```python
from build123d import *

# Parameters (mm, degrees)
SKETCH2_R           = 2.65
BOSS_EXTRUDE1_DEPTH = 2
SKETCH3_R           = 4
BOSS_EXTRUDE2_DEPTH = 10


with BuildPart() as part:
    # Sketch2 → Boss-Extrude1 (new body)
    with BuildSketch(Plane(origin=(0, 0, 0), x_dir=(1, 0, 0), z_dir=(0, 1, 0))):
        with Locations(Location((0, 0, 0), (0, 0, 270))):
            Circle(SKETCH2_R)
    extrude(amount=BOSS_EXTRUDE1_DEPTH)

    # Sketch3 → Boss-Extrude2 (add)
    with BuildSketch(Plane(origin=(0, 2, 0), x_dir=(1, 0, 0), z_dir=(0, 1, 0))):
        with Locations(Location((0, 0, 0), (0, 0, 270))):
            Circle(SKETCH3_R)
    extrude(amount=BOSS_EXTRUDE2_DEPTH)

    # Sketch4 → Cut-Loft1 section 0
    with BuildSketch(Plane.XY.offset(4)):
        with BuildLine():
            Line((-1.5, -12.39924767), (1.5, -12.39924767))
            Line((1.5, -12.39924767), (1.5, 12.39924767))
            Line((1.5, 12.39924767), (-1.5, 12.39924767))
            Line((-1.5, 12.39924767), (-1.5, -12.39924767))
        make_face()
    # Sketch5 → Cut-Loft1 section 1
    with BuildSketch(Plane.XY):
        with BuildLine():
            Line((-1, -12.21483131), (1, -12.21483131))
            Line((1, -12.21483131), (1, 12.21483131))
            Line((1, 12.21483131), (-1, 12.21483131))
            Line((-1, 12.21483131), (-1, -12.21483131))
        make_face()
    loft(mode=Mode.SUBTRACT)


solid = part.part
```
Model file for the job. Use its own axes, mm. Give positions to 0.01 mm unless a question says otherwise; leave off trailing zeros. Order: outer loops, then holes, each group sorted by start corner. A loop starts at its lowest first (then second) coordinate and runs counter-clockwise, first axis right, second up.
1) Saw through at B-B, the plane z = -1. Write the cut outline in (x, y), then the cut area to 3 significant figures.
2) Pin check, flat tip, straight feed: pin 1 (4 mm diameter, centred on x = -0.5, y = 10.5, fed in from -Z). Stop position of the tip, or through.
3) Wall check: probe 1 along Y at (x, z) = (1.75, 3); probe 2 along X at (y, z) = (5, -1.25); probe 3 along Z at (x, y) = (-0.75, 4.5). Give the ranges that are in metal, low to high.
4) Mould opens along X. For faces 1 (the flat face through (0, 6, 0)), 2 (the cylindrical face through (0.1, 0.99, -2.65)), 3 (the flat face through (0, 2, -3)) say: +X half, -X half, draft (parallel to the pull), parting line (faces both ways), or undercut.
5) Saw through at A-A, the plane x = 0. Write the cut outline in (y, z), then the cut area to 3 significant figures.
6) Saw through at D-D, the plane x = 3.25. Write the cut outline in (y, z), then the cut area to 3 significant figures.
7) Saw through at C-C, the plane z = -2.5. Write the cut outline in (x, y), then the cut area to 3 significant figures.
Computed:
1. outline: (-3.87, 2) - (-2.45, 2) - (-2.45, 0) - (2.45, 0) - (2.45, 2) - (3.87, 2) - (3.87, 12) - (-3.87, 12) - close
1. area: 87.3 mm2
2. pin 1: stops at z = -4
3. probe 1: y = 2 to 12
3. probe 2: x = -3.8 to 3.8
3. probe 3: z = -3.93 to 0
4. face 1: undercut
4. face 2: parting line
4. face 3: draft
5. outline: (0, -2.65) - (2, -2.65) - (2, -4) - (12, -4) - (12, 0) - (0, 0) - close
5. area: 45.3 mm2
6. outline: (2, -2.33) - (12, -2.33) - (12, 2.33) - (2, 2.33) - close
6. area: 46.6 mm2
7. outline: (-3.12, 2) - (-0.88, 2) - (-0.88, 0) - (0.88, 0) - (0.88, 2) - (3.12, 2) - (3.12, 12) - (-3.12, 12) - close
7. area: 66.0 mm2
